from build123d import *

# Parameters (mm, degrees)
SKETCH1_W           = 6
SKETCH1_H           = 12.1
BOSS_EXTRUDE1_DEPTH = 5
SKETCH2_R           = 2.5
BOSS_EXTRUDE2_DEPTH = 2
SKETCH4_W           = 0.8
SKETCH4_H           = 1.5
BOSS_EXTRUDE3_DEPTH = 2.8
SKETCH5_R           = 0.75
BOSS_EXTRUDE4_DEPTH = 1
SKETCH6_R           = 1.55
CUT_EXTRUDE1_DEPTH  = 10


with BuildPart() as part:
    # Sketch1 → Boss-Extrude1 (new body)
    with BuildSketch(Plane(origin=(0, 0, 0), x_dir=(1, 0, 0), z_dir=(0, 1, 0))):
        Rectangle(SKETCH1_W, SKETCH1_H)
    extrude(amount=BOSS_EXTRUDE1_DEPTH)

    # Sketch2 → Boss-Extrude2 (add)
    with BuildSketch(Plane.XY.offset(6.05)):
        with Locations(Location((0, 2.5, 0), (0, 0, 270))):
            Circle(SKETCH2_R)
    extrude(amount=BOSS_EXTRUDE2_DEPTH)

    # Sketch4 → Boss-Extrude3 (add)
    with BuildSketch(Plane.XZ):
        with Locations((2.2, 2.75)):
            Rectangle(SKETCH4_W, SKETCH4_H)
        with Locations((2.2, -0.25)):
            Rectangle(SKETCH4_W, SKETCH4_H)
        with Locations((2.2, -4.25)):
            Rectangle(SKETCH4_W, SKETCH4_H)
        with Locations((-2.2, -5.55)):
            Rectangle(SKETCH4_W, SKETCH4_H)
    extrude(amount=BOSS_EXTRUDE3_DEPTH)

    # Sketch5 → Boss-Extrude4 (add)
    with BuildSketch(Plane.XZ):
        with Locations(Location((0, 4.55, 0), (0, 0, 90))):
            Circle(SKETCH5_R)
        with Locations(Location((0, -2.45, 0), (0, 0, 90))):
            Circle(SKETCH5_R)
    extrude(amount=BOSS_EXTRUDE4_DEPTH)

    # Sketch6 → Cut-Extrude1 (cut)
    with BuildSketch(Plane.XY.offset(8.05)):
        with Locations((0, 2.5)):
            Circle(SKETCH6_R)
    extrude(amount=-CUT_EXTRUDE1_DEPTH, mode=Mode.SUBTRACT)


solid = part.part
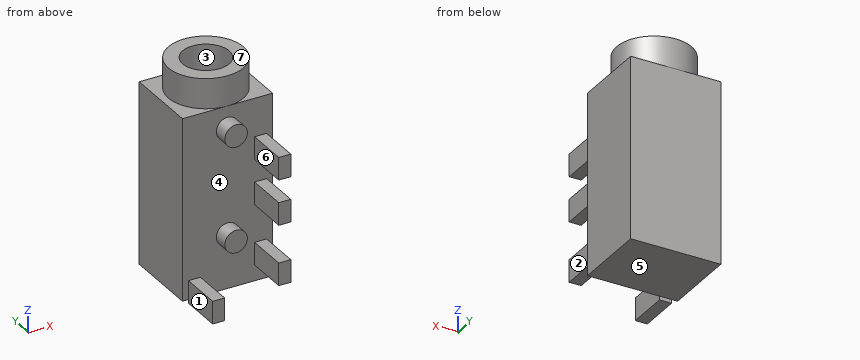
Could you check a few things on this model? Use its own coordinates, in mm. Face numbers are marked on the shaded views. A direction names the side the tool comes from. Round coordinates to 2 decimals unless told otherwise and drop trailing zeros. Order: outer loops, then holes, each group sorted by start corner. A loop starts at its lowest first (then second) coordinate and runs counter-clockwise, first axis right, second up.
Q1. Imagine slicing it at B-B, the plane z = -2.45. List the corners of the cut face in (x, y) for me.
Geometry says:
outline: (-3, 0) - (-0.75, 0) - (-0.75, -1) - (0.75, -1) - (0.75, 0) - (3, 0) - (3, 5) - (-3, 5) - close
Q2. Thinking about a two-plate mould opening in Z: for the marked faces 4, 5, 6 and 7, which applies, released by +Z, released by -Z, zero draft, split by the parting line, or undercut?
Geometry says:
face 4: undercut
face 5: released by -Z
face 6: zero draft
face 7: released by +Z
Q3. Please list where these lines run through material, in increasing order: probe 1 along Z at (x, y) = (2.45, -0.5); probe 2 along Y at (x, z) = (0, 4); probe 3 along Z at (x, y) = (2.05, 4.5).
Geometry says:
probe 1: z = -5 to -3.5, -1 to 0.5, 2 to 3.5
probe 2: y = -1 to 0.95, 4.05 to 5
probe 3: z = -6.05 to 6.05
Q4. I'm going to push flat-ended pins straight in: P1, Ø1.6, axis at y = -1, z = 3, coming from the +X side; P2, Ø0.9, axis at x = 2, y = -1.5, coming from the -Z side; P3, Ø0.9, axis at x = -2.5, y = -1, coming from the +Z side; P4, Ø2.5, axis at x = -1, y = 2.5, coming from the +Z side. Where does each tip first touch, or does it pass through?
Geometry says:
P1: stops at x = 2.6
P2: stops at z = -5
P3: stops at z = -4.8
P4: stops at z = 8.05
Q5. Imagine slicing it at C-C, the plane z = 1.75. List the corners of the cut face in (x, y) for me, then the cut area to 3 significant figures.
Geometry says:
outline: (-3, 0) - (3, 0) - (3, 5) - (-3, 5) - close; hole circle Ø3.1 at (0, 2.5)
area: 22.5 mm2
Q6. Imagine slicing it at D-D, the plane x = 1.05. List the corners of the cut face in (y, z) for me, then the cut area to 3 significant figures.
Geometry says:
outline: (0, -6.05) - (5, -6.05) - (5, 6.05) - (4.77, 6.05) - (4.77, 8.05) - (3.64, 8.05) - (3.64, -1.95) - (1.36, -1.95) - (1.36, 8.05) - (0.23, 8.05) - (0.23, 6.05) - (0, 6.05) - close
area: 46.8 mm2
Q7. Imagine slicing it at A-A, the plane y = 2.5. List the corners of the cut face in (x, z) for me, then the cut area to 3 significant figures.
Geometry says:
outline: (-3, -6.05) - (3, -6.05) - (3, 6.05) - (2.5, 6.05) - (2.5, 8.05) - (1.55, 8.05) - (1.55, -1.95) - (-1.55, -1.95) - (-1.55, 8.05) - (-2.5, 8.05) - (-2.5, 6.05) - (-3, 6.05) - close
area: 51.6 mm2
Q8. Which directions (+Z, -Z, +X, -X, +Y, -Y) give clear straight access to the entire face, cutting with the end or side of a thin tool? Please do the marked faces 1, 2 and 3.
Geometry says:
face 1: +Z, -Z, -X, -Y
face 2: +Z, -Z, +X, -Y
face 3: +Z
